The listing builds one solid part. Answer for the finished solid, in the listing's coordinates (mm). A direction names the side the tool comes from. Round coordinates to 2 decimals unless told otherwise and drop trailing zeros. Loops run counter-clockwise (first coordinate to the right, second up) from the corner with the lowest first, then second, coordinate; pieces in that order, holes last. Notation, with made-up numbers: (-2.75, 60.5) - (10.25, 60.5) arc R19 ccw to (10.25, 85.5) - close; hole circle Ø8 at (83, 33.25). An arc over 180 degrees is marked (long way). Write item = value, one per line. Start each with the question number.
1) A tool of negligible diameter and unlimited length cuts with its end or side. For faces 1 (the flat face through (-4, -2, -10)), 2 (the cylindrical face through (7.63, 2.4, -0.14)), from which of +Z, -Z, +X, -X, +Y, -Y can it reach the whole face along a straight path? Write none if from no direction.
2) Section B-B, the plane y = -117.5 is taken. Determine the outline of the cut face in (x, z), and give its area (3 significant figures).
3) Straight lines are drawn through the part: line 1 along Y through (x, z) = (-45.5, 1.25); line 2 along Z through (x, y) = (-13, -58); line 3 along Z through (x, y) = (-7, 6). For each, find the intervals that lie inside material, in ascending order.
4) For a pull along Y with two mould halves and no side action, classify faces 3 (the flat face through (-23, 21, 1)), 4 (the flat face through (-16.726, 25.211, 4.944)), 5 (the cylindrical face through (-22.37, -101.54, -5.06)) as released by +Y, released by -Y, zero draft, split by the parting line, or undercut.
5) Given pin 1 Ø6 at (x, y) = (-30.5, -85.5) entering from -Z; pin 2 Ø5 at (x, y) = (-13, 3.5) entering from -Z; pin 3 Ø5 at (x, y) = (0, 0) entering from -Z; pin 4 Ø5 at (x, y) = (-39, 45.5) entering from -Z, each flat-ended and moving along its own axis, determine where each tip first touches the part or whether it passes through.
6) Section C-C, the plane y = -53 is taken. Determine the outline of the cut face in (x, z), and give its area (3 significant figures).
7) Section A-A, the plane z = 4 is taken. Determine the outline of the cut face in (x, y).
from build123d import *

# Parameters (mm, degrees)
SKETCH_1_R        = 8
SKETCH_1_R_2      = 4
EXTRUDE_1_DEPTH   = 10
EXTRUDE_1_2_DEPTH = 10
EXTRUDE_START     = 1
EXTRUDE_2_DEPTH   = 8
EXTRUDE_START_2   = -9
EXTRUDE_3_DEPTH   = 8
EXTRUDE_START_3   = -10
SKETCH_4_R        = 8
SKETCH_4_R_2      = 4
EXTRUDE_4_DEPTH   = 10


with BuildPart() as part:
    # Sketch 1 → Extrude 1 (new body)
    with BuildSketch(Plane.XY):
        Circle(SKETCH_1_R)
        Circle(SKETCH_1_R_2, mode=Mode.SUBTRACT)
    extrude(amount=EXTRUDE_1_DEPTH)



with BuildPart() as body_2:
    # Sketch 1 → Extrude 1 2 (new body)
    with BuildSketch(Plane.XY):
        with Locations((-42.426406871, 42.426406871)):
            Circle(SKETCH_1_R)
        with Locations((-42.426406871, 42.426406871)):
            Circle(SKETCH_1_R_2, mode=Mode.SUBTRACT)
    extrude(amount=EXTRUDE_1_2_DEPTH)


with BuildPart() as part_1:
    add(part.part)

    add(body_2.part)  # Extrude 2 merges body 2
    # Sketch 2 → Extrude 2 (add)
    with BuildSketch(Plane.XY.offset(EXTRUDE_START)):
        with BuildLine():
            Line((-42.927390172, 34.442108797), (-7.984298074, -0.5009833))
            ThreePointArc((-7.984298074, -0.5009833), (-5.656854249, 5.656854249), (0.5009833, 7.984298074))
            Line((0.5009833, 7.984298074), (-34.442108797, 42.927390172))
            ThreePointArc((-34.442108797, 42.927390172), (-36.769552622, 36.769552622), (-42.927390172, 34.442108797))
        make_face()
    extrude(amount=EXTRUDE_2_DEPTH)



with BuildPart() as body_2_2:
    # Sketch 3 → Extrude 3 (new body)
    with BuildSketch(Plane.XY.offset(EXTRUDE_START_2)):
        with BuildLine():
            Line((-8, 0), (-8, -22))
            ThreePointArc((-8, -22), (-10.566583087, -42.101391623), (-18.101648629, -60.912985951))
            ThreePointArc((-18.101648629, -60.912985951), (-32.710853992, -102.552801732), (-32.548897818, -146.680762367))
            ThreePointArc((-32.548897818, -146.680762367), (-25.342004787, -151.498702844), (-20.844170391, -144.087809285))
            ThreePointArc((-20.844170391, -144.087809285), (-22.250809754, -100.941256341), (-4.418535572, -61.626962976))
            ThreePointArc((-4.418535572, -61.626962976), (4.810597012, -44.37728268), (8, -25.075571172))
            Line((8, -25.075571172), (8, 0))
            ThreePointArc((8, 0), (0, -8), (-8, 0))
        make_face()
    extrude(amount=EXTRUDE_3_DEPTH)


with BuildPart() as part_2:
    add(part_1.part)

    add(body_2_2.part)  # Extrude 4 merges body 2 2
    # Sketch 4 → Extrude 4 (add)
    with BuildSketch(Plane.XY.offset(EXTRUDE_START_3)):
        Circle(SKETCH_4_R)
        Circle(SKETCH_4_R_2, mode=Mode.SUBTRACT)
    extrude(amount=EXTRUDE_4_DEPTH)


solid = part_2.part
Geometry check:
q1.face_1 = -Z, +X, -X, +Y, -Y
q1.face_2 = none
q2.outline = (-34.35, -9) - (-24.06, -9) - (-24.06, -1) - (-34.35, -1) - close
q2.area = 82.3 mm2
q3.line_1 = 35.04 to 39.87, 44.99 to 49.81
q3.line_2 = -9 to -1
q3.line_3 = 1 to 9
q4.face_3 = zero draft
q4.face_4 = released by +Y
q4.face_5 = undercut
q5.pin_1 = -9
q5.pin_2 = 1
q5.pin_3 = through
q5.pin_4 = 0
q6.outline = (-14.25, -9) - (1.11, -9) - (1.11, -1) - (-14.25, -1) - close
q6.area = 123 mm2
q7.outline = (-42.93, 34.44) - (-7.98, -0.5) arc R8 ccw (long way) to (0.5, 7.98) - (-34.44, 42.93) arc R8 ccw (long way) to start; hole circle Ø8 at (-42.43, 42.43); hole circle Ø8 at (0, 0)
